Part model, mm, in its own coordinate system. A direction names the side the tool comes from. Coordinates: 2 decimals unless noted, no trailing zeros. Write each loop counter-clockwise with the first axis right and the second up, starting at its lowest first coordinate (ties: lowest second). Pieces come first, ordered by that corner, then holes. Notation, with made-up numbers: (7.5, 45.5) - (29.5, 45.5) arc R19 ccw to (29.5, 67.5) - close; hole circle Ø7 at (63.25, 54.5). An arc over 180 degrees is marked (long way). Use a Markdown table: item, result.
```python
from build123d import *

# Parameters (mm, degrees)
BOSS_EXTRUDE1_DEPTH = 70
SKETCH2_R           = 25
CUT_EXTRUDE1_DEPTH  = 10
SKETCH5_R           = 25
CUT_EXTRUDE3_DEPTH  = 300


with BuildPart() as part:
    # Sketch1 → Boss-Extrude1 (new body)
    with BuildSketch(Plane(origin=(0, 0, 0), x_dir=(0, 0, -1), z_dir=(1, 0, 0))):
        Polygon((-227.48711306, 131.339745962), (0, 0), (-262.679491924, 0), (-262.679491924, -10), (37.320508076, -10), (-222.48711306, 140), align=None)
    extrude(amount=BOSS_EXTRUDE1_DEPTH)

    # Sketch2 → Cut-Extrude1 (cut)
    with BuildSketch(Plane(origin=(0, 8.660254038, -5), x_dir=(1, 0, 0), z_dir=(0, 0.8660254037844418, -0.49999999999999445))):
        with Locations(Location((35, -162.679491924, 0), (0, 0, 270))):
            Circle(SKETCH2_R)
    extrude(amount=-CUT_EXTRUDE1_DEPTH, mode=Mode.SUBTRACT)

    # Sketch5 → Cut-Extrude3 (cut)
    with BuildSketch(Plane(origin=(0, 0, 0), x_dir=(1, 0, 0), z_dir=(0, 1, 0))):
        with Locations(Location((35, -202.679491924, 0), (0, 0, 270))):
            Circle(SKETCH5_R)
    extrude(amount=-CUT_EXTRUDE3_DEPTH, mode=Mode.SUBTRACT)


solid = part.part
```
Item 1: Band-saw the part on D-D, the plane z = 208. Give the cut face in (x, y).
From the geometry:
| item | result |
|---|---|
| outline | (0, -10) - (10.57, -10) - (10.57, 0) - (0, 0) - close; (0, 120.09) - (70, 120.09) - (70, 131.64) - (0, 131.64) - close; (59.43, -10) - (70, -10) - (70, 0) - (59.43, 0) - close |
Item 2: Two-plate mould, pull along Y, no slides. Class faces 3 (the face through (42.509, -4.93, 226.525)), 4 (the face through (35, -10, 115)), 5 (the face through (19.788, 75.811, 121.168)): pulls with the +Y half, pulls with the -Y half, needs draft (parallel to the pull), parting line crosses it, or undercut.
From the geometry:
| item | result |
|---|---|
| face 3 | needs draft |
| face 4 | pulls with the -Y half |
| face 5 | undercut |
Item 3: Drop flat-ended pins along their axis: P1, Ø4, axis at x = 54, y = 113, coming from the -Z side; P2, Ø3, axis at x = 31, z = 106.5, coming from the +Y side; P3, Ø4, axis at x = 10.5, y = 103.5, coming from the +Z side. Give the stop position or say it passes through.
From the geometry:
| item | result |
|---|---|
| P1 | z = 172.26 |
| P2 | y = 73.9 |
| P3 | z = 182.73 |
Item 4: Which spindle directions (+Z, -Z, +X, -X, +Y, -Y) get a long thin tool onto all of the face, cutting with end or side? Do faces 1 (the face through (0, -1, 113)), 2 (the face through (34.51, 66.59, 115.34)). Say none if no direction does.
From the geometry:
| item | result |
|---|---|
| face 1 | +Z, -Z, -X, +Y, -Y |
| face 2 | +Z, +X, -X |
Item 5: Band-saw the part on A-A, the plane z = 52.5. Give the cut face in (x, y), then the cut area to 3 significant figures.
From the geometry:
| item | result |
|---|---|
| outline | (0, -10) - (70, -10) - (70, 0) - (0, 0) - close; (0, 30.31) - (70, 30.31) - (70, 41.86) - (0, 41.86) - close |
| area | 1,510 mm^2 |
Item 6: Band-saw the part on C-C, the plane x = 6. Give the cut face in (y, z), then the cut area to 3 significant figures.
From the geometry:
| item | result |
|---|---|
| outline | (-10, -37.32) - (140, 222.49) - (131.34, 227.49) - (0, 0) - (0, 262.68) - (-10, 262.68) - close |
| area | 5,630 mm^2 |
Item 7: Band-saw the part on B-B, the plane x = 25.5. Give the cut face in (y, z), then the cut area to 3 significant figures.
From the geometry:
| item | result |
|---|---|
| outline | (-10, -37.32) - (78.44, 115.86) - (69.78, 120.86) - (0, 0) - (0, 179.55) - (-10, 179.55) - close; (-10, 225.8) - (0, 225.8) - (0, 262.68) - (-10, 262.68) - close; (92.9, 160.91) - (101.56, 155.91) - (140, 222.49) - (131.34, 227.49) - close |
| area | 4,700 mm^2 |
Item 8: Drill centre lines: probe 1 along Y at (x, z) = (13, 142.5); probe 2 along Y at (x, z) = (36.5, 33); probe 3 along Y at (x, z) = (7, 48.5). Where is each one in solid material? Low to high.
From the geometry:
| item | result |
|---|---|
| probe 1 | -10 to 0 |
| probe 2 | -10 to 0, 19.05 to 30.6 |
| probe 3 | -10 to 0, 28 to 39.55 |
